from build123d import *

# Parameters (mm, degrees)
F0_W      = 7
F0_H      = 3
F1_DEPTH  = 4
F5_W      = 7
F5_H      = 5
F6_DEPTH  = 25
F9_DEPTH  = 25
F12_DEPTH = 25
F15_W     = 10.8853101265
F15_H     = 4.9926914508
F16_DEPTH = 25
F2_W      = 0.4919341039
F2_H      = 0.3611877114
F18_DEPTH = 1
F25_DEPTH = 25


with BuildPart() as f1:
    # F0 (on Top) → F1 (new body)
    with BuildSketch(Plane.XY):
        with Locations((3.5, 1.5)):
            Rectangle(F0_W, F0_H)
    extrude(amount=F1_DEPTH)

    # F5 (on 3pt) → F6 (cut)
    with BuildSketch(Plane(origin=(0, 0, 0), x_dir=(-1, 0, 0), z_dir=(0, 0.8, -0.6))):
        with Locations((-3.5, 2.5)):
            Rectangle(F5_W, F5_H)
    extrude(amount=-F6_DEPTH, mode=Mode.SUBTRACT)

    # F8 (on 3pt) → F9 (cut)
    with BuildSketch(Plane(origin=(5.4, -1.8, 0), x_dir=(-0.316227766, -0.9486832981, 0), z_dir=(-0.9486832981, 0.316227766, 0))):
        Polygon((-1.8973665961, 0), (-5.0596442563, 4), (-5.0596442563, 1), (-5.0596442563, 0), align=None)
    extrude(amount=-F9_DEPTH, mode=Mode.SUBTRACT)

    # F11 (on 3pt) → F12 (cut)
    with BuildSketch(Plane(origin=(0, 0, 0), x_dir=(0, -1, 0), z_dir=(-0.9701425001, 0, 0.242535625))):
        Polygon((0, 0), (-3, 4.1231056256), (-3, 0), align=None)
    extrude(amount=F12_DEPTH, mode=Mode.SUBTRACT)

    # F15 (on 3pt) → F16 (cut)
    with BuildSketch(Plane(origin=(0, 0, 0), x_dir=(1, 0, 0), z_dir=(0, -0.316227766, 0.9486832981))):
        with Locations((3.1432170654, 1.333998458)):
            Rectangle(F15_W, F15_H)
    extrude(amount=-F16_DEPTH, mode=Mode.SUBTRACT)

    # F20 (on 3pt) → F21 section 0
    with BuildSketch(Plane(origin=(0, 0.4705882353, -0.1176470588), x_dir=(1, 0, 0), z_dir=(0, -0.9701425001, 0.242535625)), mode=Mode.PRIVATE) as f21_s0:
        Polygon((3, 2.1828206253), (0.25, 1.1520442189), (6.25, 1.1520442189), align=None)
    loft([f21_s0.sketch, Vertex(1, 3, 4)])

    # F23 (on 3pt) → F24 section 0
    with BuildSketch(Plane(origin=(0.08, -0.56, 0.4), x_dir=(-0.9933109617, -0.0939618477, 0.0671156055), z_dir=(-0.1154700538, 0.8082903769, -0.5773502692)), mode=Mode.PRIVATE) as f24_s0:
        Polygon((-6.211549291, 1.2496621165), (-2.9396635218, 2.2087051361), (-6.9665998531, 4.998648466), align=None)
    loft([f24_s0.sketch, Vertex(1, 3, 4)])


with BuildPart() as f18:
    # F2 (on face) → F18 (new body)
    with BuildSketch(Plane.XZ):
        with Locations((2.7540329481, 2.1805938557)):
            Rectangle(F2_W, F2_H)
    extrude(amount=F18_DEPTH)

    # F25 (cut): a face of the model
    f25_faces = [f18.faces().sort_by_distance(p)[0] for p in [
        (2.7540329481, 0, 2.1805938557),
    ]]
    extrude(f25_faces, amount=-F25_DEPTH, mode=Mode.SUBTRACT)


solid = f1.part
Check sheet for the modelled part. Datum: model origin and axes. Units: mm. Coordinates: 2 decimals unless noted, no trailing zeros. Loops run counter-clockwise (first coordinate to the right, second up) from the corner with the lowest first, then second, coordinate; pieces in that order, holes last. Notation, with made-up numbers: (27, -7) -> (49, -7) arc R8 ccw to (49, 3) -> close; hole circle Ø1 at (38.5, -32.5). An arc over 180 degrees is marked (long way). Answer in a Markdown table with one row per item.
1. Go/stop test with flat-tipped pins: pin 1 (1 mm diameter, centred on x = 4, y = 2, fed in from +Z); pin 2 (1.5 mm diameter, centred on x = 2.5, y = 1.5, fed in from -Z). Record where each tip stops, or that it passes through.
Check values:
| item | result |
|---|---|
| pin 1 | stops at z = 3.5 |
| pin 2 | stops at z = 0.25 |
2. Release check for a two-part mould opening along X. For faces 1 (the face through (5.594, 1.631, 2.365)), 2 (the face through (4, 2, 3)), 3 (the face through (0.428, 1.951, 1.713)) record: released by +X, released by -X, zero draft, split by the parting line, or undercut.
Check values:
| item | result |
|---|---|
| face 1 | released by +X |
| face 2 | zero draft |
| face 3 | released by -X |
3. Sectioned sample at B-B, the plane x = 4.25. Record the boundary of the cut face in (y, z) (3 decimals), then the cut area to 3 significant figures.
Check values:
| item | result |
|---|---|
| outline | (0, 0) -> (3, 1) -> (3, 4) -> (1.625, 2.625) -> (0.904, 1.615) -> (0.75, 1) -> close |
| area | 5.16 mm2 |
4. Sectioned sample at D-D, the plane z = 0.45. Record the boundary of the cut face in (x, y).
Check values:
| item | result |
|---|---|
| outline | (0.11, 0.34) -> (6.11, 0.34) -> (6.45, 1.35) -> (0.11, 1.35) -> close |
5. Material ranges on line 1 along Y through (x, z) = (6.25, 2.75); line 2 along Z through (x, y) = (1.5, 1.95); line 3 along Z through (x, y) = (1.5, 1.7), recorded low to high. Write a range as [from, to].
Check values:
| item | result |
|---|---|
| line 1 | y = [2, 3] |
| line 2 | z = [0.65, 2.81] |
| line 3 | z = [0.57, 2.5] |
6. Sectioned sample at C-C, the plane y = 0.25. Record the boundary of the cut face in (x, z).
Check values:
| item | result |
|---|---|
| outline | (0.02, 0.08) -> (6.08, 0.08) -> (6.08, 0.33) -> (0.08, 0.33) -> close |
7. Sectioned sample at A-A, the plane z = 1.2. Record the boundary of the cut face in (x, y), then the cut area to 3 significant figures.
Check values:
| item | result |
|---|---|
| outline | (0.3, 0.9) -> (0.8, 0.8) -> (5.6, 0.8) -> (6.3, 0.9) -> (7, 3) -> (0.3, 3) -> close |
| area | 13.9 mm2 |
